from build123d import *

# Parameters (mm, degrees)
SKETCH1_W                      = 141
SKETCH1_H                      = 161
BOSS_EXTRUDE1_DEPTH            = 5
CUT_EXTRUDE1_REACH             = 7
SKETCH2_R                      = 11.25
CUT_EXTRUDE1_DIRECTION_2_DEPTH = 1
CUT_EXTRUDE2_REACH             = 7
SKETCH3_W                      = 4
SKETCH3_H                      = 40
SKETCH4_W                      = 5
SKETCH4_H                      = 10
BOSS_EXTRUDE2_DEPTH            = 10
SKETCH5_R                      = 2.25
CUT_EXTRUDE3_DEPTH             = 4.1
CUT_EXTRUDE3_DEPTH_BACK        = 138.9
CUT_EXTRUDE4_DEPTH             = 3
CHAMFER1_SIZE                  = 3
MIRROR4_COPY_1_DEPTH           = 3
CUT_EXTRUDE5_REACH             = 17
SKETCH7_R                      = 5
SKETCH7_W                      = 20
SKETCH7_H                      = 13
CUT_EXTRUDE5_DIRECTION_2_DEPTH = 1
SKETCH8_W                      = 3.5
SKETCH8_H                      = 1
CUT_EXTRUDE6_DEPTH             = 11
CUT_EXTRUDE6_DEPTH_BACK        = 4
CUT_EXTRUDE7_REACH             = 17
SKETCH9_W                      = 14
SKETCH9_H                      = 6
CUT_EXTRUDE7_DIRECTION_2_DEPTH = 1


with BuildPart() as part:
    # Sketch1 → Boss-Extrude1 (new body)
    with BuildSketch(Plane(origin=(0, 0, 0), x_dir=(1, 0, 0), z_dir=(0, 1, 0))):
        Rectangle(SKETCH1_W, SKETCH1_H)
    extrude(amount=BOSS_EXTRUDE1_DEPTH)

    # Sketch2 → Cut-Extrude1 (cut, up to next)
    with BuildSketch(Plane(origin=(0, 5, 0), x_dir=(1, 0, 0), z_dir=(0, 1, 0)), mode=Mode.PRIVATE) as cut_extrude1_sk1:
        with Locations((50.5, 43.5)):
            Circle(SKETCH2_R)
    cut_extrude1_tool1 = extrude(cut_extrude1_sk1.sketch, amount=-CUT_EXTRUDE1_REACH, mode=Mode.PRIVATE) & part.part
    add(cut_extrude1_tool1.solids().sort_by_distance((50.5, 5, -43.5))[0], mode=Mode.SUBTRACT)

    # Sketch2 → Cut-Extrude1 direction 2 (cut)
    with BuildSketch(Plane(origin=(0, 5, 0), x_dir=(1, 0, 0), z_dir=(0, 1, 0))):
        with Locations((50.5, 43.5)):
            Circle(SKETCH2_R)
    extrude(amount=CUT_EXTRUDE1_DIRECTION_2_DEPTH, mode=Mode.SUBTRACT)

    # Sketch3 → Cut-Extrude2 (cut, up to next)
    with BuildSketch(Plane(origin=(0, 5, 0), x_dir=(1, 0, 0), z_dir=(0, 1, 0)), mode=Mode.PRIVATE) as cut_extrude2_sk1:
        with Locations((40.5, -5.5)):
            Rectangle(SKETCH3_W, SKETCH3_H)
    cut_extrude2_tool1 = extrude(cut_extrude2_sk1.sketch, amount=-CUT_EXTRUDE2_REACH, mode=Mode.PRIVATE) & part.part
    add(cut_extrude2_tool1.solids().sort_by_distance((40.5, 5, 5.5))[0], mode=Mode.SUBTRACT)
    # Sketch3 → Cut-Extrude2 (cut, up to next)
    with BuildSketch(Plane(origin=(0, 5, 0), x_dir=(1, 0, 0), z_dir=(0, 1, 0)), mode=Mode.PRIVATE) as cut_extrude2_sk2:
        with Locations((32.5, -5.5)):
            Rectangle(SKETCH3_W, SKETCH3_H)
    cut_extrude2_tool2 = extrude(cut_extrude2_sk2.sketch, amount=-CUT_EXTRUDE2_REACH, mode=Mode.PRIVATE) & part.part
    add(cut_extrude2_tool2.solids().sort_by_distance((32.5, 5, 5.5))[0], mode=Mode.SUBTRACT)
    # Sketch3 → Cut-Extrude2 (cut, up to next)
    with BuildSketch(Plane(origin=(0, 5, 0), x_dir=(1, 0, 0), z_dir=(0, 1, 0)), mode=Mode.PRIVATE) as cut_extrude2_sk3:
        with Locations((48.5, -5.5)):
            Rectangle(SKETCH3_W, SKETCH3_H)
    cut_extrude2_tool3 = extrude(cut_extrude2_sk3.sketch, amount=-CUT_EXTRUDE2_REACH, mode=Mode.PRIVATE) & part.part
    add(cut_extrude2_tool3.solids().sort_by_distance((48.5, 5, 5.5))[0], mode=Mode.SUBTRACT)
    # Sketch3 → Cut-Extrude2 (cut, up to next)
    with BuildSketch(Plane(origin=(0, 5, 0), x_dir=(1, 0, 0), z_dir=(0, 1, 0)), mode=Mode.PRIVATE) as cut_extrude2_sk4:
        with Locations((56.5, -5.5)):
            Rectangle(SKETCH3_W, SKETCH3_H)
    cut_extrude2_tool4 = extrude(cut_extrude2_sk4.sketch, amount=-CUT_EXTRUDE2_REACH, mode=Mode.PRIVATE) & part.part
    add(cut_extrude2_tool4.solids().sort_by_distance((56.5, 5, 5.5))[0], mode=Mode.SUBTRACT)
    # Sketch3 → Cut-Extrude2 (cut, up to next)
    with BuildSketch(Plane(origin=(0, 5, 0), x_dir=(1, 0, 0), z_dir=(0, 1, 0)), mode=Mode.PRIVATE) as cut_extrude2_sk5:
        with Locations((64.5, -5.5)):
            Rectangle(SKETCH3_W, SKETCH3_H)
    cut_extrude2_tool5 = extrude(cut_extrude2_sk5.sketch, amount=-CUT_EXTRUDE2_REACH, mode=Mode.PRIVATE) & part.part
    add(cut_extrude2_tool5.solids().sort_by_distance((64.5, 5, 5.5))[0], mode=Mode.SUBTRACT)

    # Sketch4 → Boss-Extrude2 (add)
    with BuildSketch(Plane.XZ):
        with Locations((64.9, 72.4)):
            Rectangle(SKETCH4_W, SKETCH4_H)
        with Locations((-64.9, 72.4)):
            Rectangle(SKETCH4_W, SKETCH4_H)
        with Locations((64.9, -72.4)):
            Rectangle(SKETCH4_W, SKETCH4_H)
        with Locations((-64.9, -72.4)):
            Rectangle(SKETCH4_W, SKETCH4_H)
    extrude(amount=BOSS_EXTRUDE2_DEPTH)

    # Sketch5 → Cut-Extrude3 (cut, two sides)
    with BuildSketch(Plane(origin=(67.4, 0, 0), x_dir=(0, 0, -1), z_dir=(1, 0, 0))) as cut_extrude3_sk:
        with Locations((-72.4, -5)):
            Circle(SKETCH5_R)
        with Locations((72.4, -5)):
            Circle(SKETCH5_R)
    extrude(amount=CUT_EXTRUDE3_DEPTH, mode=Mode.SUBTRACT)
    extrude(cut_extrude3_sk.sketch, amount=-CUT_EXTRUDE3_DEPTH_BACK, mode=Mode.SUBTRACT)

    # Sketch6 → Cut-Extrude4 (cut)
    with BuildSketch(Plane(origin=(-62.4, 0, 0), x_dir=(0, 0, -1), z_dir=(1, 0, 0))):
        Polygon((-68.185343035, -5), (-70.292671517, -1.35), (-74.507328483, -1.35), (-76.614656965, -5), (-74.507328483, -8.65), (-70.292671517, -8.65), align=None)
    cut_extrude4 = extrude(amount=-CUT_EXTRUDE4_DEPTH, mode=Mode.SUBTRACT)

    # Chamfer1
    chamfer1_edges = [part.edges().sort_by_distance(p)[0] for p in [
        (-64.9, -10, 77.4),
        (-64.9, -10, 67.4),
        (64.9, -10, -77.4),
        (64.9, -10, -67.4),
        (-64.9, -10, -77.4),
        (-64.9, -10, -67.4),
        (64.9, -10, 67.4),
        (64.9, -10, 77.4),
    ]]
    chamfer(chamfer1_edges, length=CHAMFER1_SIZE)

    # Mirror3: Cut-Extrude4 across plane
    add(cut_extrude4.mirror(Plane(origin=(0, 0, 0), x_dir=(0, 0, 1), z_dir=(1, 0, 0))), mode=Mode.SUBTRACT)

    # Mirror4: Cut-Extrude4 across plane
    add(cut_extrude4.mirror(Plane.XY), mode=Mode.SUBTRACT)

    # Mirror4 copy 1 sketch → Mirror4 copy 1 (cut)
    with BuildSketch(Plane.ZY.offset(-62.4)):
        Polygon((-68.185343035, -5), (-70.292671517, -1.35), (-74.507328483, -1.35), (-76.614656965, -5), (-74.507328483, -8.65), (-70.292671517, -8.65), align=None)
    extrude(amount=-MIRROR4_COPY_1_DEPTH, mode=Mode.SUBTRACT)

    # Sketch7 → Cut-Extrude5 (cut, up to next)
    with BuildSketch(Plane(origin=(0, 5, 0), x_dir=(1, 0, 0), z_dir=(0, 1, 0)), mode=Mode.PRIVATE) as cut_extrude5_sk1:
        with Locations((-40.5, -60.5)):
            Circle(SKETCH7_R)
    cut_extrude5_tool1 = extrude(cut_extrude5_sk1.sketch, amount=-CUT_EXTRUDE5_REACH, mode=Mode.PRIVATE) & part.part
    add(cut_extrude5_tool1.solids().sort_by_distance((-40.5, 5, 60.5))[0], mode=Mode.SUBTRACT)
    # Sketch7 → Cut-Extrude5 (cut, up to next)
    with BuildSketch(Plane(origin=(0, 5, 0), x_dir=(1, 0, 0), z_dir=(0, 1, 0)), mode=Mode.PRIVATE) as cut_extrude5_sk2:
        with Locations((-10.5, -60.5)):
            Rectangle(SKETCH7_W, SKETCH7_H)
    cut_extrude5_tool2 = extrude(cut_extrude5_sk2.sketch, amount=-CUT_EXTRUDE5_REACH, mode=Mode.PRIVATE) & part.part
    add(cut_extrude5_tool2.solids().sort_by_distance((-10.5, 5, 60.5))[0], mode=Mode.SUBTRACT)

    # Sketch7 → Cut-Extrude5 direction 2 (cut)
    with BuildSketch(Plane(origin=(0, 5, 0), x_dir=(1, 0, 0), z_dir=(0, 1, 0))):
        with Locations((-40.5, -60.5)):
            Circle(SKETCH7_R)
        with Locations((-10.5, -60.5)):
            Rectangle(SKETCH7_W, SKETCH7_H)
    extrude(amount=CUT_EXTRUDE5_DIRECTION_2_DEPTH, mode=Mode.SUBTRACT)

    # Sketch8 → Cut-Extrude6 (cut, two sides)
    with BuildSketch(Plane.XZ) as cut_extrude6_sk:
        with Locations((-40.5, 74)):
            Rectangle(SKETCH8_W, SKETCH8_H)
        with Locations((-40.5, 47)):
            Rectangle(SKETCH8_W, SKETCH8_H)
    extrude(amount=CUT_EXTRUDE6_DEPTH, mode=Mode.SUBTRACT)
    extrude(cut_extrude6_sk.sketch, amount=-CUT_EXTRUDE6_DEPTH_BACK, mode=Mode.SUBTRACT)

    # Sketch9 → Cut-Extrude7 (cut, up to next)
    with BuildSketch(Plane(origin=(0, 5, 0), x_dir=(1, 0, 0), z_dir=(0, 1, 0)), mode=Mode.PRIVATE) as cut_extrude7_sk1:
        with Locations((0, 77.5)):
            Rectangle(SKETCH9_W, SKETCH9_H)
    cut_extrude7_tool1 = extrude(cut_extrude7_sk1.sketch, amount=-CUT_EXTRUDE7_REACH, mode=Mode.PRIVATE) & part.part
    add(cut_extrude7_tool1.solids().sort_by_distance((0, 5, -77.5))[0], mode=Mode.SUBTRACT)

    # Sketch9 → Cut-Extrude7 direction 2 (cut)
    with BuildSketch(Plane(origin=(0, 5, 0), x_dir=(1, 0, 0), z_dir=(0, 1, 0))):
        with Locations((0, 77.5)):
            Rectangle(SKETCH9_W, SKETCH9_H)
    extrude(amount=CUT_EXTRUDE7_DIRECTION_2_DEPTH, mode=Mode.SUBTRACT)


solid = part.part
Geometry: final body of the model. Coordinates: model frame, mm. A direction names the side the tool comes from. Give positions to 0.01 mm unless a question says otherwise; leave off trailing zeros. Order: outer loops, then holes, each group sorted by start corner. A loop starts at its lowest first (then second) coordinate and runs counter-clockwise, first axis right, second up. Notation, with made-up numbers: (48.25, -28) - (80.25, -28) arc R16 ccw to (80.25, -23) - close; hole circle Ø11 at (51, -18.75). An arc over 180 degrees is marked (long way). Use CSV: the item, a comma, the result in double quotes.
1. Contact query for flat-ended pins moving along their axis: pin 1 (4 mm diameter, centred on x = -53.5, z = 63, fed in from -Y); pin 2 (0.8 mm diameter, centred on x = -41, z = 47, fed in from -Y); pin 3 (5 mm diameter, centred on y = -3.5, z = -71, fed in from +X); pin 4 (1.5 mm diameter, centred on y = -2, z = 51.5, fed in from +X). Output: stop coordinate, or through.
Answers below:
pin 1,"y = 0"
pin 2,"y = 4"
pin 3,"x = 67.4"
pin 4,"through"
2. Section query A-A (z = 3). Output: boundary loops of the cut face in (x, y), plus the area to 3 significant figures.
Answers below:
outline,"(-70.5, 0) - (30.5, 0) - (30.5, 5) - (-70.5, 5) - close; (34.5, 0) - (38.5, 0) - (38.5, 5) - (34.5, 5) - close; (42.5, 0) - (46.5, 0) - (46.5, 5) - (42.5, 5) - close; (50.5, 0) - (54.5, 0) - (54.5, 5) - (50.5, 5) - close; (58.5, 0) - (62.5, 0) - (62.5, 5) - (58.5, 5) - close; (66.5, 0) - (70.5, 0) - (70.5, 5) - (66.5, 5) - close"
area,"605 mm2"
3. Material intervals for line 1 along X through (y, z) = (3.25, -43.5); line 2 along Y through (x, z) = (65.95, -72.4); line 3 along Z through (x, y) = (56, 1.75), sorted ascending. Write a range as from..to.
Answers below:
line 1,"-70.5..39.25, 61.75..70.5"
line 2,"-10..-7.25, -2.75..5"
line 3,"-80.5..-53.31, -33.69..-14.5, 25.5..80.5"
4. Access query for faces 1 (the face through (-65, -3, -77.4)), 2 (the face through (-62.4, -3, 69)), 3 (the face through (48, 3, 25.5)). Directions: +Z, -Z, +X, -X, +Y, -Y. A direction counts if a zero-diameter tool reaches every point of the face in a straight line with its end or side. Return the directions, or none.
Answers below:
face 1,"-Z, +X, -X, -Y"
face 2,"+Z, -Z, -Y"
face 3,"+Y, -Y"
5. Section query C-C (z = -72.4). Output: boundary loops of the cut face in (x, y), plus the area to 3 significant figures.
Answers below:
outline,"(-70.5, 0) - (-67.4, 0) - (-67.4, -2.75) - (-65.4, -2.75) - (-65.4, -1.35) - (-62.4, -1.35) - (-62.4, 0) - (62.4, 0) - (62.4, -1.35) - (65.4, -1.35) - (65.4, -2.75) - (67.4, -2.75) - (67.4, 0) - (70.5, 0) - (70.5, 5) - (-70.5, 5) - close; (-67.4, -10) - (-62.4, -10) - (-62.4, -8.65) - (-65.4, -8.65) - (-65.4, -7.25) - (-67.4, -7.25) - close; (62.4, -10) - (67.4, -10) - (67.4, -7.25) - (65.4, -7.25) - (65.4, -8.65) - (62.4, -8.65) - close"
area,"743 mm2"
6. Section query B-B (x = -40.5). Output: boundary loops of the cut face in (y, z), plus the area to 3 significant figures.
Answers below:
outline,"(0, -80.5) - (5, -80.5) - (5, 55.5) - (0, 55.5) - (0, 47.5) - (4, 47.5) - (4, 46.5) - (0, 46.5) - close; (0, 65.5) - (5, 65.5) - (5, 80.5) - (0, 80.5) - (0, 74.5) - (4, 74.5) - (4, 73.5) - (0, 73.5) - close"
area,"747 mm2"
7. Section query D-D (x = -4). Output: boundary loops of the cut face in (y, z).
Answers below:
outline,"(0, -74.5) - (5, -74.5) - (5, 54) - (0, 54) - close; (0, 67) - (5, 67) - (5, 80.5) - (0, 80.5) - close"
8. Mould query, pull axis X, two halves, no side actions, for faces 4 (the face through (-1, 0, -1)), 5 (the face through (-70.5, 2, 1)), 6 (the face through (-65, -3, 67.4)), 7 (the face through (64, 3, -14.5)). Classes: +X half, -X half, draft (parallel to the pull), parting line (faces both ways), or undercut.
Answers below:
face 4,"undercut"
face 5,"-X half"
face 6,"draft"
face 7,"undercut"
